```python
from build123d import *

# Parameters (mm, degrees)
SKETCH1_W           = 40
SKETCH1_H           = 50
BOSS_EXTRUDE1_DEPTH = 5
BOSS_EXTRUDE2_DEPTH = 7.5
FILLET3_R           = 10
SKETCH6_W           = 36
SKETCH6_H           = 10
BOSS_EXTRUDE3_DEPTH = 18
SKETCH7_R           = 8
CUT_EXTRUDE3_DEPTH  = 5
FILLET5_R           = 5
SKETCH8_R           = 1.6
CUT_EXTRUDE4_DEPTH  = 100.116132934
FILLET6_R           = 3
BOSS_EXTRUDE4_DEPTH = 15
SKETCH10_R          = 1
CUT_EXTRUDE5_DEPTH  = 500.756658462
FILLET8_R           = 10
FILLET9_R           = 7
CUT_EXTRUDE7_DEPTH  = 5
FILLET10_R          = 4
SKETCH13_W          = 10
SKETCH13_H          = 6
BOSS_EXTRUDE5_DEPTH = 25
CHAMFER1_SIZE       = 8
FILLET11_R          = 5
FILLET12_R          = 3
BOSS_EXTRUDE7_DEPTH = 10
CHAMFER2_SIZE       = 10
FILLET15_R          = 10
FILLET16_R          = 3
FILLET17_R          = 5
SKETCH19_R          = 1.25
CUT_EXTRUDE8_DEPTH  = 10
SKETCH20_R          = 2.5
CUT_EXTRUDE9_DEPTH  = 153.367653519


with BuildPart() as part:
    # Sketch1 → Boss-Extrude1 (new body)
    with BuildSketch(Plane.XY):
        with Locations((0, 421.657979857)):
            Rectangle(SKETCH1_W, SKETCH1_H)
    extrude(amount=BOSS_EXTRUDE1_DEPTH)

    # Sketch5 → Boss-Extrude2 (add, symmetric)
    with BuildSketch(Plane(origin=(0, 0, 0), x_dir=(0, 0, -1), z_dir=(1, 0, 0))):
        Polygon((-10, 370), (-10, 467.320715151), (16, 467.320715151), (42.019504932, 422.253610621), (76.24600224, 422.253610621), (76.24600224, 412.253610621), (36.24600224, 412.253610621), (10.226497308, 457.320715151), (0, 457.320715151), (0, 370), align=None)
    extrude(amount=BOSS_EXTRUDE2_DEPTH, both=True)

    # Fillet3
    fillet3_edges = [part.edges().sort_by_distance(p)[0] for p in [
        (0, 457.320715151, -10.226497308),
        (0, 412.253610621, -36.24600224),
        (0, 422.253610621, -42.019504932),
        (0, 467.320715151, 10),
    ]]
    fillet(fillet3_edges, radius=FILLET3_R)

    # Sketch6 → Boss-Extrude3 (add, symmetric)
    with BuildSketch(Plane(origin=(0, 0, 0), x_dir=(0, 0, -1), z_dir=(1, 0, 0))):
        with Locations((63.814228499, 417.253610621)):
            Rectangle(SKETCH6_W, SKETCH6_H)
    extrude(amount=BOSS_EXTRUDE3_DEPTH, both=True)

    # Sketch7 → Cut-Extrude3 (cut)
    with BuildSketch(Plane(origin=(0, 422.253610621, 0), x_dir=(1, 0, 0), z_dir=(0, 1, 0))):
        with Locations(Location((0, 63.814228499, 0), (0, 0, 270))):
            Circle(SKETCH7_R)
    extrude(amount=-CUT_EXTRUDE3_DEPTH, mode=Mode.SUBTRACT)

    # Fillet5
    fillet5_edges = [part.edges().sort_by_distance(p)[0] for p in [
        (-7.5, 417.253610621, -45.814228499),
    ]]
    fillet(fillet5_edges, radius=FILLET5_R)
    fillet5_2_edges = [part.edges().sort_by_distance(p)[0] for p in [
        (-18, 417.253610621, -45.814228499),
    ]]
    fillet(fillet5_2_edges, radius=FILLET5_R)
    fillet5_3_edges = [part.edges().sort_by_distance(p)[0] for p in [
        (7.5, 417.253610621, -45.814228499),
    ]]
    fillet(fillet5_3_edges, radius=FILLET5_R)
    fillet5_4_edges = [part.edges().sort_by_distance(p)[0] for p in [
        (18, 417.253610621, -45.814228499),
    ]]
    fillet(fillet5_4_edges, radius=FILLET5_R)
    fillet5_5_edges = [part.edges().sort_by_distance(p)[0] for p in [
        (18, 417.253610621, -81.814228499),
    ]]
    fillet(fillet5_5_edges, radius=FILLET5_R)
    fillet5_6_edges = [part.edges().sort_by_distance(p)[0] for p in [
        (-18, 417.253610621, -81.814228499),
    ]]
    fillet(fillet5_6_edges, radius=FILLET5_R)

    # Sketch8 → Cut-Extrude4 (cut, through all)
    with BuildSketch(Plane(origin=(0, 422.253610621, 0), x_dir=(1, 0, 0), z_dir=(0, 1, 0))):
        with Locations(Location((11.66726189, 52.14696661, 0), (0, 0, 270))):
            Circle(SKETCH8_R)
        with Locations(Location((-11.66726189, 52.14696661, 0), (0, 0, 270))):
            Circle(SKETCH8_R)
        with Locations(Location((-11.66726189, 75.481490389, 0), (0, 0, 270))):
            Circle(SKETCH8_R)
        with Locations(Location((11.66726189, 75.481490389, 0), (0, 0, 270))):
            Circle(SKETCH8_R)
    extrude(amount=-CUT_EXTRUDE4_DEPTH, mode=Mode.SUBTRACT)

    # Fillet6
    fillet6_edges = [part.edges().sort_by_distance(p)[0] for p in [
        (-20, 446.657979857, 2.5),
        (20, 446.657979857, 2.5),
        (20, 396.657979857, 2.5),
        (-20, 396.657979857, 2.5),
    ]]
    fillet(fillet6_edges, radius=FILLET6_R)

    # Sketch9 → Boss-Extrude4 (add)
    with BuildSketch(Plane(origin=(7.5, 0, 0), x_dir=(0, 0, -1), z_dir=(1, 0, 0))):
        Polygon((26, 450.000207075), (26, 495.000207075), (16, 495.000207075), (16, 467.320715151), align=None)
    extrude(amount=-BOSS_EXTRUDE4_DEPTH)

    # Sketch10 → Cut-Extrude5 (cut, through all)
    with BuildSketch(Plane.XY.offset(-16)):
        with Locations((0, 491.000207075)):
            Circle(SKETCH10_R)
    extrude(amount=-CUT_EXTRUDE5_DEPTH, mode=Mode.SUBTRACT)

    # Fillet8
    fillet8_edges = [part.edges().sort_by_distance(p)[0] for p in [
        (0, 450.000207075, -26),
    ]]
    fillet(fillet8_edges, radius=FILLET8_R)

    # Fillet9
    fillet9_edges = [part.edges().sort_by_distance(p)[0] for p in [
        (7.5, 495.000207075, -21),
        (-7.5, 495.000207075, -21),
    ]]
    fillet(fillet9_edges, radius=FILLET9_R)

    # Sketch12 → Cut-Extrude7 (cut)
    with BuildSketch(Plane.XY.offset(5)):
        with BuildLine():
            Line((7.5, 396.657979857), (17, 396.657979857))
            ThreePointArc((17, 396.657979857), (19.121320344, 397.536659513), (20, 399.657979857))
            Line((20, 399.657979857), (20, 443.657979857))
            ThreePointArc((20, 443.657979857), (19.121320344, 445.7793002), (17, 446.657979857))
            Line((17, 446.657979857), (7.5, 446.657979857))
            Line((7.5, 446.657979857), (7.5, 396.657979857))
        make_face()
        with BuildLine():
            Line((-20, 443.657979857), (-20, 399.657979857))
            ThreePointArc((-20, 399.657979857), (-19.121320344, 397.536659513), (-17, 396.657979857))
            Line((-17, 396.657979857), (-7.5, 396.657979857))
            Line((-7.5, 396.657979857), (-7.5, 446.657979857))
            Line((-7.5, 446.657979857), (-17, 446.657979857))
            ThreePointArc((-17, 446.657979857), (-19.121320344, 445.7793002), (-20, 443.657979857))
        make_face()
    extrude(amount=-CUT_EXTRUDE7_DEPTH, mode=Mode.SUBTRACT)

    # Fillet10
    fillet10_edges = [part.edges().sort_by_distance(p)[0] for p in [
        (0, 457.320715151, 0),
    ]]
    fillet(fillet10_edges, radius=FILLET10_R)

    # Sketch13 → Boss-Extrude5 (add, symmetric)
    with BuildSketch(Plane(origin=(0, 0, 0), x_dir=(0, 0, -1), z_dir=(1, 0, 0))):
        with Locations((-5, 373)):
            Rectangle(SKETCH13_W, SKETCH13_H)
    extrude(amount=BOSS_EXTRUDE5_DEPTH, both=True)

    # Chamfer1
    chamfer1_edges = [part.edges().sort_by_distance(p)[0] for p in [
        (7.5, 376, 5),
        (-7.5, 376, 5),
    ]]
    chamfer(chamfer1_edges, length=CHAMFER1_SIZE)

    # Fillet11
    fillet11_edges = [part.edges().sort_by_distance(p)[0] for p in [
        (-15.5, 376, 5),
        (-7.5, 384, 5),
        (7.5, 384, 5),
        (15.5, 376, 5),
    ]]
    fillet(fillet11_edges, radius=FILLET11_R)

    # Fillet12
    fillet12_edges = [part.edges().sort_by_distance(p)[0] for p in [
        (-25, 373, 10),
        (-25, 373, 0),
        (25, 373, 10),
        (25, 373, 0),
    ]]
    fillet(fillet12_edges, radius=FILLET12_R)

    # Sketch18 → Boss-Extrude7 (add)
    with BuildSketch(Plane(origin=(0, 0, -81.814228499), x_dir=(-1, 0, 0), z_dir=(0, 0, -1))):
        with BuildLine():
            Line((7.5, 412.253610621), (7.5, 488.000207075))
            ThreePointArc((7.5, 488.000207075), (5.449747468, 492.949954543), (0.5, 495.000207075))
            Line((0.5, 495.000207075), (-0.5, 495.000207075))
            ThreePointArc((-0.5, 495.000207075), (-5.449747468, 492.949954543), (-7.5, 488.000207075))
            Line((-7.5, 488.000207075), (-7.5, 412.253610621))
            Line((-7.5, 412.253610621), (7.5, 412.253610621))
        make_face()
    extrude(amount=BOSS_EXTRUDE7_DEPTH)

    # Chamfer2
    chamfer2_edges = [part.edges().sort_by_distance(p)[0] for p in [
        (0, 412.253610621, -91.814228499),
    ]]
    chamfer(chamfer2_edges, length=CHAMFER2_SIZE)

    # Fillet15
    fillet15_edges = [part.edges().sort_by_distance(p)[0] for p in [
        (0, 422.253610621, -91.814228499),
    ]]
    fillet(fillet15_edges, radius=FILLET15_R)

    # Fillet16
    fillet16_edges = [part.edges().sort_by_distance(p)[0] for p in [
        (0, 422.253610621, -81.814228499),
    ]]
    fillet(fillet16_edges, radius=FILLET16_R)

    # Fillet17
    fillet17_edges = [part.edges().sort_by_distance(p)[0] for p in [
        (7.5, 417.253610621, -81.814228499),
        (-7.5, 417.253610621, -81.814228499),
    ]]
    fillet(fillet17_edges, radius=FILLET17_R)

    # Sketch19 → Cut-Extrude8 (cut)
    with BuildSketch(Plane(origin=(0, 0, -91.814228499), x_dir=(-1, 0, 0), z_dir=(0, 0, -1))):
        with Locations(Location((0, 491.000207075, 0), (0, 0, 90))):
            Circle(SKETCH19_R)
    extrude(amount=-CUT_EXTRUDE8_DEPTH, mode=Mode.SUBTRACT)

    # Sketch20 → Cut-Extrude9 (cut, through all)
    with BuildSketch(Plane(origin=(0, 376, 0), x_dir=(1, 0, 0), z_dir=(0, 1, 0))):
        with Locations(Location((-20, -5, 0), (0, 0, 270))):
            Circle(SKETCH20_R)
        with Locations(Location((20, -5, 0), (0, 0, 270))):
            Circle(SKETCH20_R)
    extrude(amount=-CUT_EXTRUDE9_DEPTH, mode=Mode.SUBTRACT)


solid = part.part
```
Can you work these out from the model? Positions are in its coordinate system, mm. A direction names the side the tool comes from. Give positions to 0.01 mm unless a question says otherwise; leave off trailing zeros. Order: outer loops, then holes, each group sorted by start corner. A loop starts at its lowest first (then second) coordinate and runs counter-clockwise, first axis right, second up. Notation, with made-up numbers: (-28.5, -22) - (-8.5, -22) arc R14 cw to (-8.5, -9) - close; hole circle Ø9 at (68.5, -10.5). An arc over 180 degrees is marked (long way). Use a Markdown table: item, result. Add a question column.
Q1. If we mould it in two halves opening along X, with no side actions, what happens to faces 4 (the flat face through (7.5, 453, -87)), 5 (the cylindrical face through (-5.4, 493, -20.9)), 6 (the cylindrical face through (11.74, 417.32, -77.08)), 7 (the flat face through (8.3, 422.254, -63.5))? For each: released by +X, released by -X, zero draft, split by the parting line, or undercut.
Q2. Please list where these lines run through material, in increasing order: line 1 along Z through (x, y) = (2, 476.5); line 2 along Z through (x, y) = (-20, 373.5); line 3 along X through (y, z) = (454, -25.5).
Q3. On a 3-axis mill with a long thin cutter (end or side, diameter ignored), from which of +Z, -Z, +X, -X, +Y, -Y can I reach the whole of each face in a straight line? I mean faces 1 (the flat face through (23, 376, 5)), 2 (the flat face through (0.1, 434.5, -23.4)), 3 (the cylindrical face through (-0.1, 423.2, -81)). Say none if no direction works.
Q4. If we section it at A-A on x = -20: Write out the boundary of the cut face in (y, z).
Q5. I'm going to push flat-ended pins straight in: pin 1 (16.5 mm diameter, centred on x = 1, z = -6, fed in from +Y); pin 2 (1 mm diameter, centred on x = -9, z = -46.5, fed in from -Y); pin 3 (21 mm diameter, centred on x = 0, z = -63.81, fed in from +Y); pin 4 (10 mm diameter, centred on y = 437.5, z = -43, fed in from -X). Where does each tip first touch, or does it pass through?
Q6. If we section it at B-B on y = 397.5: Write out the boundary of the cut face in (x, z), plus the area to 3 significant figures.
Answers follow:
| question | item | result |
|---|---|---|
| 1 | face 4 | released by +X |
| 1 | face 5 | released by -X |
| 1 | face 6 | undercut |
| 1 | face 7 | zero draft |
| 2 | line 1 | z = -91.81 to -81.81, -26 to -16 |
| 2 | line 2 | z = 0 to 2.5, 7.5 to 10 |
| 2 | line 3 | x = -7.5 to 7.5 |
| 3 | face 1 | +Z, -Z, +X, +Y |
| 3 | face 2 | +X, -X, -Y |
| 3 | face 3 | +X, -X, +Y |
| 4 | outline | (370, 0) - (376, 0) - (376, 2.5) - (370, 2.5) - close; (370, 7.5) - (376, 7.5) - (376, 10) - (370, 10) - close |
| 5 | pin 1 | stops at y = 467.32 |
| 5 | pin 2 | stops at y = 412.25 |
| 5 | pin 3 | stops at y = 422.25 |
| 5 | pin 4 | passes through |
| 6 | outline | (-7.5, 0) - (7.5, 0) - (7.5, 10) - (-7.5, 10) - close |
| 6 | area | 150 mm^2 |
